from build123d import *

# Parameters (mm, degrees)
SKETCH_W        = 4.72
SKETCH_H        = 5.2
PAD_DEPTH       = 15
POCKET_DEPTH    = 38.001
POCKET005_DEPTH = 12
SKETCH003_R     = 1.5
POCKET006_DEPTH = 5
FILLET_R        = 1.99
FILLET001_R     = 10
FILLET002_R     = 5
SKETCH004_W     = 5
SKETCH004_H     = 4.23039
POCKET007_DEPTH = 6


with BuildPart() as part:
    # Sketch → Pad (new body)
    with BuildSketch(Plane.XY):
        Polygon((-19, 19), (-19, -19), (19, -19), (19, 19), (17, 19), (17, 26.7), (6, 26.7), (6, 19), (-6, 19), (-6, 26.7), (-17, 26.7), (-17, 19), align=None)
        with Locations((-12.41, 21.6)):
            Rectangle(SKETCH_W, SKETCH_H, mode=Mode.SUBTRACT)
        with Locations((12.41, 21.6)):
            Rectangle(SKETCH_W, SKETCH_H, mode=Mode.SUBTRACT)
    extrude(amount=PAD_DEPTH)

    # Sketch001 (on Face3 of Pad) → Pocket (cut, through all)
    with BuildSketch(Plane.YZ.offset(19)):
        Polygon((26.7, 8), (26.7, 0), (3.7, 0), (11.7, 8), align=None)
    extrude(amount=-POCKET_DEPTH, mode=Mode.SUBTRACT)

    # Sketch002 (on Face6 of Pocket) → Pocket005 (cut)
    with BuildSketch(Plane.XY.offset(15)):
        Polygon((-9.25, -19), (9.25, -19), (9.25, 6.35), (6, 6.35), (6, 19), (-6, 19), (-6, 6.35), (-9.25, 6.35), align=None)
    extrude(amount=-POCKET005_DEPTH, mode=Mode.SUBTRACT)

    # Sketch003 → Pocket006 (cut)
    with BuildSketch(Plane.XY.offset(4)):
        with Locations((-5.25, -5.15)):
            Circle(SKETCH003_R)
        with Locations((5.25, -5.15)):
            Circle(SKETCH003_R)
    extrude(amount=-POCKET006_DEPTH, mode=Mode.SUBTRACT)

    # Fillet
    fillet_edges = [part.edges().sort_by_distance(p)[0] for p in [
        (17, 26.7, 11.5),
        (6, 26.7, 11.5),
        (-6, 26.7, 11.5),
        (-17, 26.7, 11.5),
        (-19, 19, 11.5),
        (19, 19, 11.5),
        (19, -19, 7.5),
        (-19, -19, 7.5),
    ]]
    fillet(fillet_edges, radius=FILLET_R)

    # Fillet001
    fillet001_edges = [part.edges().sort_by_distance(p)[0] for p in [
        (0, 3.7, 0),
    ]]
    fillet(fillet001_edges, radius=FILLET001_R)

    # Fillet002
    fillet002_edges = [part.edges().sort_by_distance(p)[0] for p in [
        (12.5, 11.7, 8),
        (-12.5, 11.7, 8),
    ]]
    fillet(fillet002_edges, radius=FILLET002_R)

    # Sketch004 (on Face10 of Fillet002) → Pocket007 (cut)
    with BuildSketch(Plane.YZ.offset(19)):
        with Locations((2.7, 2.115195)):
            Rectangle(SKETCH004_W, SKETCH004_H)
    extrude(amount=-POCKET007_DEPTH, mode=Mode.SUBTRACT)


solid = part.part
Can you work these out from the model? Positions are in its coordinate system, mm. A direction names the side the tool comes from. Round coordinates to 2 decimals unless told otherwise and drop trailing zeros. Loops run counter-clockwise (first coordinate to the right, second up) from the corner with the lowest first, then second, coordinate; pieces in that order, holes last. Notation, with made-up numbers: (58.5, -3) - (117.5, -3) arc R29 cw to (117.5, 29) - close; hole circle Ø3 at (78, 18). An arc over 180 degrees is marked (long way). Write item = value, one per line. Start each with the question number.
(1) If we section it at B-B (x = 5.25): Please give me the cut outline in (y, z), and give its area (3 significant figures).
(2) If we section it at A-A (z = 13.75): Give the number of separate pieces and of enclosed holes in the cut face, and give its area (3 significant figures).
(3) For faces 1 (the face through (16, 0.2, 2)), 2 (the face through (-10.05, 22, 11)), 3 (the face through (12.6, 18.7, 8)), which set-ups out of +Z, -Z, +X, -X, +Y, -Y let a thin tool reach every point of the face, with its end or its side?
(4) If we mould it in two halves opening along X, with no side actions, what happens to faces 4 (the face through (18.402, -18.433, 7.605)), 5 (the face through (-18.433, -18.402, 7.605)), 6 (the face through (12, 19, 11))? For each: released by +X, released by -X, zero draft, split by the parting line, or undercut.
(5) If we section it at D-D (y = -5.15): Please give me the cut outline in (x, z), and give its area (3 significant figures).
(6) If I drill on probe 1 along X at (y, z) = (-12, 10.75); probe 2 along Y at (x, z) = (11, 11); probe 3 along Z at (x, y) = (-8.5, 16), over which ranges is the centre line in solid material (lowest first)? Write a range as [from, to].
(7) If we section it at C-C (y = 23): Please give me the cut outline in (x, z), and give its area (3 significant figures).
(8) For P1, Ø14, axis at x = -10, y = 19, coming from the -Z side; P2, Ø8, axis at x = 9.5, y = 5.5, coming from the -Z side; P3, Ø12, axis at x = 4, y = 18.5, coming from the -Z side, each with a flat end and sliding along its axis, tell me the tip position at first contact or that it passes through.
Ans:
q1.outline = (-19, 0) - (-6.65, 0) - (-6.65, 3) - (-19, 3) - close; (-3.65, 0) - (-0.44, 0) arc R10 ccw to (6.63, 2.93) - (6.7, 3) - (-3.65, 3) - close
q1.area = 61.4 mm²
q2.separate_pieces = 2
q2.enclosed_holes = 2
q2.area = 937 mm²
q3.face_1 = -Z, +X
q3.face_2 = +Z, -Z
q3.face_3 = -Z, +X, -X, +Y
q4.face_4 = released by +X
q4.face_5 = released by -X
q4.face_6 = undercut
q5.outline = (-19, 0) - (-6.75, 0) - (-6.75, 3) - (-9.25, 3) - (-9.25, 15) - (-19, 15) - close; (-3.75, 0) - (3.75, 0) - (3.75, 3) - (-3.75, 3) - close; (6.75, 0) - (19, 0) - (19, 15) - (9.25, 15) - (9.25, 3) - (6.75, 3) - close
q5.area = 330 mm²
q6.probe_1 = [-19, -9.25], [9.25, 19]
q6.probe_2 = [-19, 19], [24.2, 26.7]
q6.probe_3 = [8, 15]
q7.outline = (-17, 8) - (-14.77, 8) - (-14.77, 15) - (-17, 15) - close; (-10.05, 8) - (-6, 8) - (-6, 15) - (-10.05, 15) - close; (6, 8) - (10.05, 8) - (10.05, 15) - (6, 15) - close; (14.77, 8) - (17, 8) - (17, 15) - (14.77, 15) - close
q7.area = 87.9 mm²
q8.P1 = 7.68
q8.P2 = 0.19
q8.P3 = 7.91
